For this review, take the finished solid that the model builds, in its own axes (mm). A direction names the side the tool comes from. Round coordinates to 2 decimals unless told otherwise and drop trailing zeros. Write each loop counter-clockwise with the first axis right and the second up, starting at its lowest first coordinate (ties: lowest second). Pieces come first, ordered by that corner, then holes. Notation, with made-up numbers: (21, 12) -> (65, 12) arc R22 cw to (65, 30) -> close; hole circle Ø2 at (38.5, -15.75). An arc over 180 degrees is marked (long way). Answer as CSV lines item,"result". Start each with the question number.
Item 1: Take a section at B-B on x = -35. Give the boundary of the cut face in (y, z).
Item 2: For pin 1 Ø8.5 at (x, y) = (-69.5, 8) entering from -Z; pin 2 Ø1.5 at (x, y) = (39, 8) entering from +Z; pin 3 Ø12 at (x, z) = (36, 31) entering from -Y; pin 4 Ø5.5 at (y, z) = (-1, 16) entering from -X, all flat-tipped, find the tip position at first contact; note any pin that passes through.
Item 3: Take a section at C-C on y = -24.5. Give the boundary of the cut face in (x, z), then the cut area to 3 significant figures.
Item 4: Take a section at A-A on z = 15. Give the boundary of the cut face in (x, y).
Item 5: Machinability: for faces 1 (the cylindrical face through (-60.746, 30.3, 18.783)), 2 (the flat face through (-10, -25.84, 21)), 3 (the flat face through (-68.056, 12.867, 36.222)), which of the approach directions +Z, -Z, +X, -X, +Y, -Y give a long, thin tool a straight path to every point of the face, cutting with its end or side? Answer none if there is none.
Item 6: Mouldability with a two-part tool opening along Y and no side actions: class faces 4 (the cylindrical face through (57.264, -7.158, 36.222)), 5 (the flat face through (-60.895, 2, 21)), 6 (the flat face through (-69.395, 15.471, 36.222)) as +Y half, -Y half, draft (parallel to the pull), parting line (faces both ways), or undercut.
Item 7: Take a section at D-D on y = 32. Give the boundary of the cut face in (x, z), then the cut area to 3 significant figures.
Item 8: Wall thickness on probe 1 along Y at (x, z) = (1.5, 7); probe 2 along Y at (x, z) = (-42.5, 20); probe 3 along X at (y, z) = (-6, 13): over which ranges is each line inside the solid? List them lowest first. Write a range as from..to.
```python
from build123d import *

# Parameters (mm, degrees)
F1_DEPTH = 38.1
F3_DEPTH = 35.56
F5_DEPTH = 3.81


with BuildPart() as f1:
    # F0 (on Top) → F1 (new body)
    with BuildSketch(Plane.XY):
        with BuildLine():
            Line((28.9094160199, 35.7320394768), (-47.4246910334, 35.7320394768))
            ThreePointArc((-47.4246910334, 35.7320394768), (-60.895075215, 30.1524236584), (-66.4746910334, 16.6820394768))
            Line((-66.4746910334, 16.6820394768), (-66.4746910334, -12.3694256604))
            ThreePointArc((-66.4746910334, -12.3694256604), (-60.895075215, -25.839809842), (-47.4246910334, -31.4194256604))
            Line((-47.4246910334, -31.4194256604), (28.9094160199, -31.4194256604))
            ThreePointArc((28.9094160199, -31.4194256604), (42.3798002015, -25.839809842), (47.9594160199, -12.3694256604))
            Line((47.9594160199, -12.3694256604), (47.9594160199, 16.6820394768))
            ThreePointArc((47.9594160199, 16.6820394768), (42.3798002015, 30.1524236584), (28.9094160199, 35.7320394768))
        make_face()
    extrude(amount=F1_DEPTH)

    # F2 (on face) → F3 (cut)
    with BuildSketch(Plane.XY.offset(38.1)):
        with BuildLine():
            Line((23.3298002015, 30.1524236584), (-41.845075215, 30.1524236584))
            ThreePointArc((-41.845075215, 30.1524236584), (-55.3154593966, 24.57280784), (-60.895075215, 11.1024236584))
            Line((-60.895075215, 11.1024236584), (-60.895075215, -6.789809842))
            ThreePointArc((-60.895075215, -6.789809842), (-55.3154593966, -20.2601940236), (-41.845075215, -25.839809842))
            Line((-41.845075215, -25.839809842), (23.3298002015, -25.839809842))
            ThreePointArc((23.3298002015, -25.839809842), (36.8001843831, -20.2601940236), (42.3798002015, -6.789809842))
            Line((42.3798002015, -6.789809842), (42.3798002015, 11.1024236584))
            ThreePointArc((42.3798002015, 11.1024236584), (36.8001843831, 24.57280784), (23.3298002015, 30.1524236584))
        make_face()
    extrude(amount=-F3_DEPTH, mode=Mode.SUBTRACT)

    # F4 (on face) → F5 (join)
    with BuildSketch(Plane.XY.offset(38.1)):
        with BuildLine():
            Line((47.9594160199, -8.8493684307), (47.9594160199, -12.3694256604))
            Line((47.9594160199, -12.3694256604), (53.8822529313, -9.912228523))
            ThreePointArc((53.8822529313, -9.912228523), (57.2992531994, -7.1055718841), (58.5822723806, -2.87389679))
            Line((58.5822723806, -2.87389679), (58.5822723806, 7.1865106064))
            ThreePointArc((58.5822723806, 7.1865106064), (57.2992531994, 11.4181857005), (53.8822529313, 14.2248423394))
            Line((53.8822529313, 14.2248423394), (47.9594160199, 16.6820394768))
            Line((47.9594160199, 16.6820394768), (47.9594160199, 13.1619822471))
            Line((47.9594160199, 13.1619822471), (51.0777804109, 12.5797672736))
            ThreePointArc((51.0777804109, 12.5797672736), (55.5410437685, 9.9578611105), (57.2992531994, 5.0892051025))
            Line((57.2992531994, 5.0892051025), (57.2992531994, -0.7765912861))
            ThreePointArc((57.2992531994, -0.7765912861), (55.5410437685, -5.6452472941), (51.0777804109, -8.2671534572))
            Line((51.0777804109, -8.2671534572), (47.9594160199, -8.8493684307))
        make_face()
        with BuildLine():
            Line((-72.3975279448, -9.912228523), (-66.4746910334, -12.3694256604))
            Line((-66.4746910334, -12.3694256604), (-66.4746910334, -8.8493684307))
            Line((-66.4746910334, -8.8493684307), (-69.5930554243, -8.2671534572))
            ThreePointArc((-69.5930554243, -8.2671534572), (-74.0563187819, -5.6452472941), (-75.8145282129, -0.7765912861))
            Line((-75.8145282129, -0.7765912861), (-75.8145282129, 5.0892051025))
            ThreePointArc((-75.8145282129, 5.0892051025), (-74.0563187819, 9.9578611105), (-69.5930554243, 12.5797672736))
            Line((-69.5930554243, 12.5797672736), (-66.4746910334, 13.1619822471))
            Line((-66.4746910334, 13.1619822471), (-66.4746910334, 16.6820394768))
            Line((-66.4746910334, 16.6820394768), (-72.3975279448, 14.2248423394))
            ThreePointArc((-72.3975279448, 14.2248423394), (-75.8145282129, 11.4181857005), (-77.097547394, 7.1865106064))
            Line((-77.097547394, 7.1865106064), (-77.097547394, -2.87389679))
            ThreePointArc((-77.097547394, -2.87389679), (-75.8145282129, -7.1055718841), (-72.3975279448, -9.912228523))
        make_face()
    extrude(amount=-F5_DEPTH)


solid = f1.part
```
Output values:
1,outline,"(-31.42, 0) -> (35.73, 0) -> (35.73, 38.1) -> (30.15, 38.1) -> (30.15, 2.54) -> (-25.84, 2.54) -> (-25.84, 38.1) -> (-31.42, 38.1) -> close"
2,pin 1,"stops at z = 0"
2,pin 2,"stops at z = 2.54"
2,pin 3,"stops at y = -31.39"
2,pin 4,"stops at x = -66.47"
3,outline,"(-62.11, 0) -> (43.6, 0) -> (43.6, 38.1) -> (30.35, 38.1) -> (30.35, 2.54) -> (-48.86, 2.54) -> (-48.86, 38.1) -> (-62.11, 38.1) -> close"
3,area,"1,210 mm^2"
4,outline,"(-66.47, -12.37) arc R19.05 ccw to (-47.42, -31.42) -> (28.91, -31.42) arc R19.05 ccw to (47.96, -12.37) -> (47.96, 16.68) arc R19.05 ccw to (28.91, 35.73) -> (-47.42, 35.73) arc R19.05 ccw to (-66.47, 16.68) -> close; hole (-60.9, -6.79) arc R19.05 ccw to (-41.85, -25.84) -> (23.33, -25.84) arc R19.05 ccw to (42.38, -6.79) -> (42.38, 11.1) arc R19.05 ccw to (23.33, 30.15) -> (-41.85, 30.15) arc R19.05 ccw to (-60.9, 11.1) -> close"
5,face 1,"+Z, -Z, -X, +Y"
5,face 2,"+Z"
5,face 3,"+Z, -Z"
6,face 4,"-Y half"
6,face 5,"undercut"
6,face 6,"+Y half"
7,outline,"(-58.75, 0) -> (40.23, 0) -> (40.23, 38.1) -> (-58.75, 38.1) -> close"
7,area,"3,770 mm^2"
8,probe 1,"y = -31.42..-25.84, 30.15..35.73"
8,probe 2,"y = -31.42..-25.83, 30.14..35.73"
8,probe 3,"x = -66.47..-60.9, 42.38..47.96"
